Autodesk Inventor part; units mm, degrees
ref_plane "Work Plane1" through (0, 50.8, 0) normal (0, 1, 0) x (-1, 0, 0)
ref_plane "YZ Plane" through (0, 0, 0) normal (1, 0, 0) x (0, 1, 0)
ref_plane "XY Plane" through (0, 0, 0) normal (0, 0, 1) x (1, 0, 0)
sketch "Sketch6" plane through (0, 0, 0) normal (0, 1, 0) x (-1, 0, 0)
  line L0 (0, 0) -> (5.588, 0)
  line L1 (5.588, 0) -> (5.588, -6.35)
  line L2 (5.588, -6.35) -> (0, -6.35)
  line L3 (0, -6.35) -> (0, 0)
  arc A0 (0, -6.35) -> (5.588, -6.35) centre (2.794, -6.35) ccw
  dimension "d25" = 5.588
  dimension "d26" = 6.35
ref_plane "Work Plane1" through (0, 50.8, 0) normal (0, 1, 0) x (-1, 0, 0)
sketch "Sketch8" plane through (0, 50.8, 0) normal (0, 1, 0) x (-1, 0, 0)
  line L0 (4.3815, 0) -> (1.2065, 0)
  line L1 (1.2065, 0) -> (1.2065, -3.81)
  line L2 (1.2065, -3.81) -> (4.3815, -3.81)
  line L3 (4.3815, -3.81) -> (4.3815, 0)
  arc A0 (1.2065, -3.81) -> (4.3815, -3.81) centre (2.794, -3.81) ccw
  point P0 (0, 0)
  dimension "d27" = 3.175
  dimension "d28" = 3.81
  dimension "d49" = 1.2065
loft "Loft1" add profiles "Sketch6", "Sketch8"
sketch "Sketch9" plane through (-5.588, 0, 0) normal (0, 0, 1) x (1, 0, 0)
  line L0 (0, 0) -> (5.588, 0)
  line L1 (5.588, 0) -> (4.3815, 50.8)
  line L2 (1.2065, 50.8) -> (4.3815, 50.8)
  line L3 (0, 0) -> (1.2065, 50.8)
  line L4 (4.3815, 50.8) -> (5.588, 0)
  line L5 (4.5323, 44.45) -> (1.0557, 44.45)
  line L6 (0, 0) -> (1.2065, 50.8)
  dimension "d34" = 6.35
extrude "Extrusion5" add sketch "Sketch9" along normal blind 38.608 contours L3 L2 L1 L5
sketch "Sketch12" plane through (-2.794, 0, -6.35) normal (0, -1, 0) x (1, 0, 0)
  circle A0 centre (0, 1.9685) radius 1.27
  arc A1 (-2.794, 0) -> (2.794, 0) centre (0, 0) ccw
  line L0 (0, -2.794) -> (0, 1.9685)
  point P0 (2.794, 6.35)
  dimension "d44" = 2.54
  dimension "d46" = 4.7625
extrude "Extrusion8" cut sketch "Sketch12" against normal blind 10.16
sketch "Sketch13" plane through (-5.588, 0, 0) normal (0, 0, 1) x (1, 0, 0)
  line L0 (4.3815, 50.8) -> (1.2065, 50.8)
  line L1 (1.2065, 50.8) -> (4.3815, 50.8)
  line L2 (1.0557, 44.45) -> (4.5323, 44.45)
  line L3 (3.683, 50.8) -> (1.905, 50.8)
  line L4 (1.905, 50.8) -> (1.905, 44.45)
  line L5 (1.905, 44.45) -> (3.683, 44.45)
  line L6 (3.683, 44.45) -> (3.683, 50.8)
  line L7 (3.683, 50.8) -> (4.3815, 50.8) construction
  line L8 (0, 0) -> (1.2065, 50.8) construction
  line L9 (1.905, 50.8) -> (1.2065, 50.8) construction
  line L10 (6.4775, 53.5114) -> (-2.6174, 53.5114)
  line L11 (-2.6174, 53.5114) -> (-2.6174, 42.707)
  line L12 (-2.6174, 42.707) -> (6.4775, 42.707)
  line L13 (6.4775, 42.707) -> (6.4775, 53.5114)
  point P0 (5.588, 0)
  dimension "d50" = 1.778
extrude "Extrusion9" cut sketch "Sketch13" against normal through all contours L6 L2 L4 L0
extrude "Extrusion10" cut sketch "Sketch13" along normal through all contours L6 L2 L4 L0 | L13 L12 L11 L10
properties part number "RudderStabilizingFins_Print1"
Verification items for the finished model (mm, model axes). A direction names the side the tool comes from. Give positions to 0.01 mm unless a question says otherwise; leave off trailing zeros.
1. Mould release check, pull along Z, two halves, no side actions. Record for faces 3 (the flat face through (-3, 44.45, -3)), 4 (the flat face through (-3, 10.16, -4)), 5 (the flat face through (-3, 20, 0)), 6 (the cylindrical face through (-3.07, 5.01, -5.62)): released by +Z, released by -Z, zero draft, split by the parting line, or undercut.
2. Thickness scan on line 1 (Y direction, x = -2.2, z = -0.5); line 2 (X direction, y = 45, z = -1.25) (3 decimals); line 3 (X direction, y = 12.5, z = -5.75). Record the ranges inside material, lowest first.
3. Set-up check for faces 1 (the flat face through (-3, 0, -6)), 2 (the flat face through (-1.905, 48, -3)): record each of +Z, -Z, +X, -X, +Y, -Y from which the full face is reachable in a straight line by a thin tool's end or side.
4. Go/stop test with flat-tipped pins: pin 1 Ø1.7 at (y, z) = (48, -2) entering from +X; pin 2 Ø0.5 at (x, z) = (-2.5, -2.5) entering from +Y; pin 3 Ø5 at (y, z) = (44.5, -2) entering from +X. Record where each tip stops, or that it passes through.
Geometry says:
1. face 3: zero draft
1. face 4: undercut
1. face 5: released by +Z
1. face 6: undercut
2. line 1: y = 0 to 44.45
2. line 2: x = -4.519 to -3.683, -1.905 to -1.069
2. line 3: x = -5.29 to -0.3
3. face 1: +Z, -Z, +X, -X, -Y
3. face 2: +Z, -Z, +Y
4. pin 1: stops at x = -1.12
4. pin 2: stops at y = 44.45
4. pin 3: stops at x = -1
